Source: CAD feature listing. Evaluate the final solid. Frame: model axes, mm. Face numbers are marked on the shaded views. Give positions to 0.01 mm unless a question says otherwise; leave off trailing zeros. Loops run counter-clockwise (first coordinate to the right, second up) from the corner with the lowest first, then second, coordinate; pieces in that order, holes last. Notation, with made-up numbers: M 57.25,-24.75 L 76.25,-24.75 A31 ccw 76.25,13.25 Z; hole C -12.5,-10.75 d8. An arc over 180 degrees is marked long. Answer in a Markdown table with one row per item.
```python
from build123d import *

# Parameters (mm, degrees)
F0_W     = 101.6
F0_H     = 76.2
F1_DEPTH = 76.2
F2_R     = 17.309068
F3_DEPTH = 76.2


with BuildPart() as f1:
    # F0 (on Front) → F1 (new body)
    with BuildSketch(Plane.XZ):
        with Locations((50.8, 38.1)):
            Rectangle(F0_W, F0_H)
    extrude(amount=F1_DEPTH)

    # F2 (on Front) → F3 (cut, through all)
    with BuildSketch(Plane.XZ):
        with Locations((44.897694, 35.112303)):
            Circle(F2_R)
    extrude(amount=F3_DEPTH, mode=Mode.SUBTRACT)


solid = f1.part
```
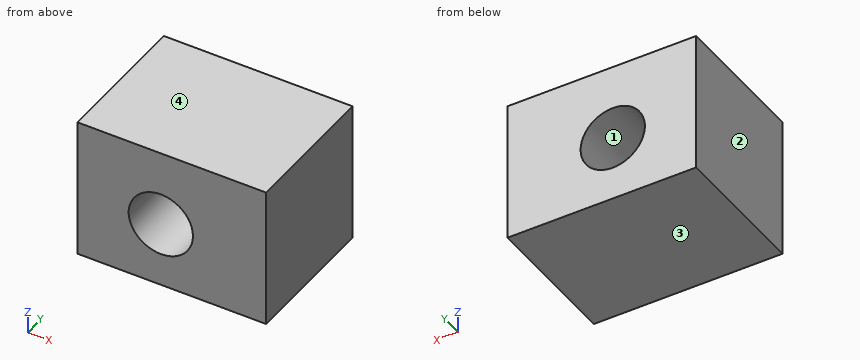
1) Pull-direction query (Z, two-part tool) for the marked faces 1, 2, 3 and 4; classes: released by +Z, released by -Z, zero draft, split by the parting line, or undercut.
Reply:
| item | result |
|---|---|
| face 1 | undercut |
| face 2 | zero draft |
| face 3 | released by -Z |
| face 4 | released by +Z |
2) Section C-C, the plane y = -68. Return loops of the section in (x, z).
Reply:
| item | result |
|---|---|
| outline | M 0,0 L 101.6,0 L 101.6,76.2 L 0,76.2 Z; hole C 44.9,35.11 d34.62 |
3) Section B-B, the plane x = 42. Return loops of the section in (y, z), then the cut area to 3 significant figures.
Reply:
| item | result |
|---|---|
| outline | M -76.2,0 L 0,0 L 0,18.05 L -76.2,18.05 Z; M -76.2,52.18 L 0,52.18 L 0,76.2 L -76.2,76.2 Z |
| area | 3,210 mm² |
4) Section A-A, the plane z = 46. Return loops of the section in (x, y).
Reply:
| item | result |
|---|---|
| outline | M 0,-76.2 L 31.44,-76.2 L 31.44,0 L 0,0 Z; M 58.35,-76.2 L 101.6,-76.2 L 101.6,0 L 58.35,0 Z |
5) Material intervals for L1, parallel to X at y = -25.5, z = 35; L2, parallel to X at y = -72.5, z = 27; L3, parallel to Z at x = 49.5, y = -27, sorted ascending.
Reply:
| item | result |
|---|---|
| L1 | x = 0 to 27.59, 62.21 to 101.6 |
| L2 | x = 0 to 29.61, 60.19 to 101.6 |
| L3 | z = 0 to 18.43, 51.8 to 76.2 |
